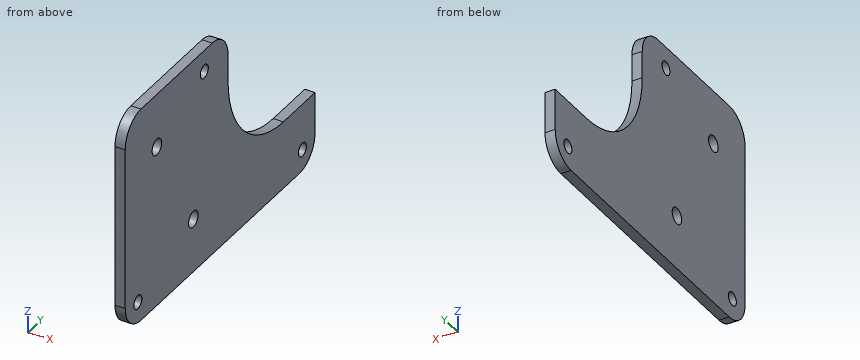
from build123d import *

# Parameters (mm, degrees)
SKETCH1_R           = 3
SKETCH1_R_2         = 2.5
BOSS_EXTRUDE1_DEPTH = 3.8
FILLET1_R           = 10


with BuildPart() as part:
    # Sketch1 → Boss-Extrude1 (new body)
    with BuildSketch(Plane(origin=(0, 0, 0), x_dir=(0, 0, -1), z_dir=(1, 0, 0))):
        with BuildLine():
            Line((-33.760087735, -70.625), (46.510087735, -70.625))
            Line((46.510087735, -70.625), (46.510087735, 49.375))
            Line((46.510087735, 49.375), (21.239912265, 49.375))
            Line((21.239912265, 49.375), (21.239912265, 29.375))
            ThreePointArc((21.239912265, 29.375), (10.988649606, 4.626262658), (-13.760087735, -5.625))
            Line((-13.760087735, -5.625), (-33.760087735, -5.625))
            Line((-33.760087735, -5.625), (-33.760087735, -70.625))
        make_face()
        with Locations((-13.760087735, -50.625)):
            Circle(SKETCH1_R, mode=Mode.SUBTRACT)
        with Locations((26.510087735, -27.575640625)):
            Circle(SKETCH1_R, mode=Mode.SUBTRACT)
        with Locations((38.510087735, 41.375)):
            Circle(SKETCH1_R_2, mode=Mode.SUBTRACT)
        with Locations((38.510087735, -62.625)):
            Circle(SKETCH1_R_2, mode=Mode.SUBTRACT)
        with Locations((-25.760087735, -20.625)):
            Circle(SKETCH1_R_2, mode=Mode.SUBTRACT)
    extrude(amount=BOSS_EXTRUDE1_DEPTH)

    # Fillet1
    fillet1_edges = [part.edges().sort_by_distance(p)[0] for p in [
        (1.9, -70.625, -46.510087735),
        (1.9, -70.625, 33.760087735),
        (1.9, -5.625, 33.760087735),
        (1.9, 49.375, -46.510087735),
    ]]
    fillet(fillet1_edges, radius=FILLET1_R)


solid = part.part
Model file for the job. Use its own axes, mm. Give positions to 0.01 mm unless a question says otherwise; leave off trailing zeros. Order: outer loops, then holes, each group sorted by start corner. A loop starts at its lowest first (then second) coordinate and runs counter-clockwise, first axis right, second up. Notation, with made-up numbers: M -5.5,8 L 24.5,8 A18 cw 24.5,24 Z; hole C -35,7.25 d4. An arc over 180 degrees is marked long. Put each result on its own line as item: value. Start each with the question number.
(1) Pin check, flat tip, straight feed: pin 1 Ø1.1 at (x, y) = (1, 37) entering from +Z. Stop position of the tip, or through.
(2) Band-saw the part on D-D on y = 25. Give the cut face in (x, z).
(3) Drill centre lines: L1, parallel to Y at x = 3.1, z = -37; L2, parallel to Y at x = 1.2, z = 26.5; L3, parallel to Z at x = 3.6, y = 29.5. Where is each one in solid material? Low to high. Write a range as [from, to].
(4) Band-saw the part on B-B on x = 1.45. Give the cut face in (y, z) (3 decimals), then the cut area to 3 significant figures.
(5) Band-saw the part on A-A on z = 25. Give the cut face in (x, y).
(6) Band-saw the part on C-C on z = -26. Give the cut face in (x, y) (3 decimals).
Results below:
1. pin 1: stops at z = -21.24
2. outline: M 0,-46.51 L 3.8,-46.51 L 3.8,-20.97 L 0,-20.97 Z
3. L1: y = [-70.61, -64.62], [-60.63, 39.38], [43.37, 49.36]
3. L2: y = [-70.24, -23.01], [-18.24, -6.01]
3. L3: z = [-46.51, -21.24]
4. outline: M -70.625,-36.51 A10 ccw -60.625,-46.51 L 39.375,-46.51 A10 ccw 49.375,-36.51 L 49.375,-21.24 L 29.375,-21.24 A35 cw -5.625,13.76 L -5.625,23.76 A10 ccw -15.625,33.76 L -60.625,33.76 A10 ccw -70.625,23.76 Z; hole C -62.625,-38.51 d5; hole C -50.625,13.76 d6; hole C -27.576,-26.51 d6; hole C -20.625,25.76 d5; hole C 41.375,-38.51 d5
4. area: 6,670 mm2
5. outline: M 0,-70.55 L 3.8,-70.55 L 3.8,-23.01 L 0,-23.01 Z; M 0,-18.24 L 3.8,-18.24 L 3.8,-5.7 L 0,-5.7 Z
6. outline: M 0,-70.625 L 3.8,-70.625 L 3.8,-30.532 L 0,-30.532 Z; M 0,-24.619 L 3.8,-24.619 L 3.8,49.375 L 0,49.375 Z
